Can you work these out from the model? Positions are in its coordinate system, mm. Round coordinates to 2 decimals unless told otherwise and drop trailing zeros. Write each loop counter-clockwise with the first axis right and the second up, starting at its lowest first coordinate (ties: lowest second). Pieces come first, ordered by that corner, then holes.
Q1. If we section it at B-B (x = -14): Please give me the cut outline in (y, z), plus the area to 3 significant figures.
Q2. If we section it at A-A (y = 8.5): Please give me the cut outline in (x, z).
Q3. Please list where these lines run through material, in increasing order: line 1 along Y through (x, z) = (-10, 0.65); line 2 along X through (y, z) = (15.75, 0.65); line 3 along Y through (x, z) = (-7.5, 0.65).
from build123d import *

# Parameters (mm, degrees)
SKETCH_1_W          = 10
SKETCH_1_H          = 10
EXTRUDE_1_DEPTH     = 0.7
SKETCH_2_W          = 10
SKETCH_2_H          = 10
CUT_EXTRUDE_1_DEPTH = 0.1
FILLET_1_R          = 0.2


with BuildPart() as part:
    # 草图1 → 凸台-拉伸1 (new body)
    with BuildSketch(Plane.XY):
        with Locations((-10.731707317, 12.731707317)):
            Rectangle(SKETCH_1_W, SKETCH_1_H)
    extrude(amount=EXTRUDE_1_DEPTH)

    # 草图2 → 切除-拉伸1 (cut)
    with BuildSketch(Plane.XY.offset(0.7)):
        with Locations((-10.731707317, 12.731707317)):
            Rectangle(SKETCH_2_W, SKETCH_2_H)
        with BuildLine():
            Line((-15.389589016, 17.419802303), (-9.02347014, 17.419802303))
            ThreePointArc((-9.02347014, 17.419802303), (-6.902149796, 16.541122647), (-6.02347014, 14.419802303))
            Line((-6.02347014, 14.419802303), (-6.02347014, 8.073825618))
            Line((-6.02347014, 8.073825618), (-12.389589016, 8.073825618))
            ThreePointArc((-12.389589016, 8.073825618), (-14.51090936, 8.952505274), (-15.389589016, 11.073825618))
            Line((-15.389589016, 11.073825618), (-15.389589016, 17.419802303))
        make_face(mode=Mode.SUBTRACT)
    extrude(amount=-CUT_EXTRUDE_1_DEPTH, mode=Mode.SUBTRACT)

    # 圆角1
    fillet_1_edges = [part.edges().sort_by_distance(p)[0] for p in [
        (-15.731707317, 17.731707317, 0.3),
        (-5.731707317, 17.731707317, 0.3),
        (-5.731707317, 7.731707317, 0.3),
        (-15.731707317, 7.731707317, 0.3),
    ]]
    fillet(fillet_1_edges, radius=FILLET_1_R)


solid = part.part
A:
1. outline: (7.73, 0) - (17.73, 0) - (17.73, 0.6) - (17.42, 0.6) - (17.42, 0.7) - (8.54, 0.7) - (8.54, 0.6) - (7.73, 0.6) - close
1. area: 6.89 mm2
2. outline: (-15.73, 0) - (-5.73, 0) - (-5.73, 0.6) - (-6.02, 0.6) - (-6.02, 0.7) - (-13.93, 0.7) - (-13.93, 0.6) - (-15.73, 0.6) - close
3. line 1: y = 8.07 to 17.42
3. line 2: x = -15.39 to -6.33
3. line 3: y = 8.07 to 17
